Can you work these out from the model? Positions are in its coordinate system, mm. Round coordinates to 2 decimals unless told otherwise and drop trailing zeros. Write each loop counter-clockwise with the first axis right and the second up, starting at its lowest first coordinate (ties: lowest second). Pieces come first, ordered by that corner, then holes. Notation, with made-up numbers: M 30,80.25 L 55,80.25 A11 cw 55,100.25 Z; hole C 47.5,56.25 d7. An arc over 180 degrees is marked long. Answer in a Markdown table with one row per item. Add a question column.
(1) If we mould it in two halves opening along Y, with no side actions, what happens to faces 1 (the face through (29.9, 9.4, 0.5)), 2 (the face through (31.73, 9.99, 19.46)), 3 (the face through (14, -29, -20))? For each: released by +Y, released by -Y, zero draft, split by the parting line, or undercut.
(2) I'm going to push flat-ended pins straight in: pin 1 (2 mm diameter, centred on y = 18.5, z = -2.5, fed in from +X); pin 2 (10 mm diameter, centred on y = -46, z = 1, fed in from +X); pin 3 (10 mm diameter, centred on x = 49.5, y = 41.5, fed in from +Z). Where does each tip first touch, or does it pass through?
(3) Suppose I cut it at A-A, the plane z = 12. Write out the boundary of the cut face in (x, y), then the cut area to 3 significant figures.
(4) If I drill on probe 1 along X at (y, z) = (-2, -7); probe 2 along Y at (x, z) = (0, 4); probe 3 along Y at (x, z) = (-11.5, -3), over which ranges is the centre line in solid material (lowest first)?
(5) Suppose I cut it at B-B, the plane z = -14. Write out the boundary of the cut face in (x, y).
from build123d import *

# Parameters (mm, degrees)
F0_R          = 75
F1_DEPTH      = 50
F1_TAPER      = 65
F1_DEPTH_BACK = 20
F1_TAPER_BACK = 20
F2_R          = 5
F3_R          = 31.3436912466
F4_DEPTH      = 50
F4_DEPTH_BACK = 25


with BuildPart() as f1:
    # F0 (on Top) → F1 (new body, two sides)
    with BuildSketch(Plane.XY) as f1_sk:
        Circle(F0_R)
    extrude(amount=F1_DEPTH, taper=F1_TAPER)
    extrude(f1_sk.sketch, amount=-F1_DEPTH_BACK, taper=F1_TAPER_BACK)

    # F2
    f2_edges = [f1.edges().sort_by_distance(p)[0] for p in [
        (-75, 0, 0),
    ]]
    fillet(f2_edges, radius=F2_R)

    # F3 (on Top) → F4 (cut, two sides)
    with BuildSketch(Plane.XY) as f4_sk:
        Circle(F3_R)
    extrude(amount=F4_DEPTH, mode=Mode.SUBTRACT)
    extrude(f4_sk.sketch, amount=-F4_DEPTH_BACK, mode=Mode.SUBTRACT)


solid = f1.part
Calculated:
| question | item | result |
|---|---|---|
| 1 | face 1 | undercut |
| 1 | face 2 | split by the parting line |
| 1 | face 3 | zero draft |
| 2 | pin 1 | x = 71.63 |
| 2 | pin 2 | x = 60.7 |
| 2 | pin 3 | z = 7.18 |
| 3 | outline | C 0,0 d98.53; hole C 0,0 d62.69 |
| 3 | area | 4,540 mm² |
| 4 | probe 1 | -72.42 to -31.28, 31.28 to 72.42 |
| 4 | probe 2 | -66.42 to -31.34, 31.34 to 66.42 |
| 4 | probe 3 | -72.82 to -29.16, 29.16 to 72.82 |
| 5 | outline | C 0,0 d139.81; hole C 0,0 d62.69 |
